Model file for the job. Use its own axes, mm. Coordinates: 2 decimals unless noted, no trailing zeros. Write each loop counter-clockwise with the first axis right and the second up, starting at its lowest first coordinate (ties: lowest second). Pieces come first, ordered by that corner, then holes. Notation, with made-up numbers: (6, -24.75) - (42, -24.75) arc R9 ccw to (42, -14.75) - close; hole circle Ø4 at (23.25, 58.5). An arc over 180 degrees is marked (long way). Put each result on its own line as item: value. Start each with the question number.
1. Drill centre lines: L1, parallel to Y at x = 19, z = 6; L2, parallel to X at y = 67, z = 4.75; L3, parallel to Y at x = 13, z = 4.75. Where is each one in solid material? Low to high. Write a range as from..to.
2. Saw through at B-B, the plane x = 34.5. Write the cut outline in (y, z).
3. Pull direction Y, two halves, no side cores. Call faces 1 (the face through (0, 126, 4)), 2 (the face through (99.57, 23.11, 3.55)), 3 (the face through (80, 0, 3)): released by +Y, released by -Y, zero draft, split by the parting line, or undercut.
4. Saw through at A-A, the plane z = 4.75. Write the cut outline in (x, y), plus the area to 3 significant figures.
5. Drop flat-ended pins along their axis: P1, Ø1.5, axis at y = 87, z = 5, coming from the +X side; P2, Ø3, axis at y = 143, z = 3, coming from the +X side. Give the stop position or say it passes through.
6. Saw through at C-C, the plane y = 98.5. Write the cut outline in (x, z), plus the area to 3 significant figures.
```python
from build123d import *

# Parameters (mm, degrees)
BOSS_EXTRUDE1_DEPTH = 7
FILLET1_R           = 33
SKETCH2_R           = 60
CUT_EXTRUDE1_DEPTH  = 259.610511066
SKETCH3_W           = 181.044086137
SKETCH3_H           = 480.78858802
CUT_EXTRUDE2_DEPTH  = 259.610511066
SKETCH4_W           = 169.768954509
SKETCH4_H           = 49.097500459
CUT_EXTRUDE3_DEPTH  = 215.823183106


with BuildPart() as part:
    # Sketch1 → Boss-Extrude1 (new body)
    with BuildSketch(Plane.XY):
        with BuildLine():
            Line((-100, 0), (100, 0))
            Line((100, 0), (100, 23.252721757))
            Line((100, 23.252721757), (26.948185903, 238.391267529))
            Line((26.948185903, 238.391267529), (24.948185903, 238.391267529))
            ThreePointArc((24.948185903, 238.391267529), (0, 215), (-24.948185903, 238.391267529))
            Line((-24.948185903, 238.391267529), (-26.948185903, 238.391267529))
            Line((-26.948185903, 238.391267529), (-100, 23.252721757))
            Line((-100, 23.252721757), (-100, 0))
        make_face()
    extrude(amount=BOSS_EXTRUDE1_DEPTH)

    # Fillet1
    fillet1_edges = [part.edges().sort_by_distance(p)[0] for p in [
        (-100, 23.252721757, 3.5),
        (100, 23.252721757, 3.5),
    ]]
    fillet(fillet1_edges, radius=FILLET1_R)

    # Sketch2 → Cut-Extrude1 (cut, through all)
    with BuildSketch(Plane.XY.offset(7)):
        Circle(SKETCH2_R)
    extrude(amount=-CUT_EXTRUDE1_DEPTH, mode=Mode.SUBTRACT)

    # Sketch3 → Cut-Extrude2 (cut, through all)
    with BuildSketch(Plane(origin=(0, 0, 0), x_dir=(0, 0, -1), z_dir=(1, 0, 0))):
        with Locations((-2.723537344, 108.130535203)):
            Rectangle(SKETCH3_W, SKETCH3_H)
    extrude(amount=-CUT_EXTRUDE2_DEPTH, mode=Mode.SUBTRACT)

    # Sketch4 → Cut-Extrude3 (cut, through all)
    with BuildSketch(Plane(origin=(0, 190, 0), x_dir=(1, 0, 0), z_dir=(0, 1, 0))):
        with Locations((45.695998337, 2.995854363)):
            Rectangle(SKETCH4_W, SKETCH4_H)
    extrude(amount=CUT_EXTRUDE3_DEPTH, mode=Mode.SUBTRACT)


solid = part.part
```
Final values:
1. L1: y = 56.91..190
1. L2: x = 0..85.15
1. L3: y = 58.57..190
2. outline: (49.09, 0) - (190, 0) - (190, 7) - (49.09, 7) - close
3. face 1: zero draft
3. face 2: released by +Y
3. face 3: released by -Y
4. outline: (0, 60) arc R60 cw to (60, 0) - (100, 0) - (100, 17.8) arc R33 ccw to (98.25, 28.41) - (43.38, 190) - (0, 190) - close
4. area: 11,500 mm²
5. P1: stops at x = 78.61
5. P2: stops at x = 59.85
6. outline: (0, 0) - (74.45, 0) - (74.45, 7) - (0, 7) - close
6. area: 521 mm²
